Autodesk Inventor part; units mm, degrees
ref_plane "YZ Plane" through (0, 0, 0) normal (1, 0, 0) x (0, 1, 0)
ref_plane "XZ Plane" through (0, 0, 0) normal (0, 1, 0) x (-1, 0, 0)
ref_plane "XY Plane" through (0, 0, 0) normal (0, 0, 1) x (1, 0, 0)
sketch "sqr_sketch" plane through (0, 0, 0) normal (1, 0, 0) x (0, 1, 0)
  line L0 (12.7, 12.7) -> (-12.7, 12.7)
  line L1 (-12.7, 12.7) -> (-12.7, -12.7)
  line L2 (-12.7, -12.7) -> (12.7, -12.7)
  line L3 (12.7, -12.7) -> (12.7, 12.7)
  line L4 (12.7, 12.7) -> (-12.7, -12.7) construction
  line L5 (-12.7, 12.7) -> (12.7, -12.7) construction
  point P0 (0, 0)
  dimension "d0" = 25.4
extrude "sqr_extrusion" add sketch "sqr_sketch" along normal mid plane 25.4
sketch "T_sketch" plane through (-12.7, -12.7, 12.7) normal (0, 0, 1) x (1, 0, 0)
  line L0 (5.5534, 21.59) -> (19.8466, 21.59) construction
  line L1 (19.8466, 21.59) -> (19.8466, 3.81) construction
  line L2 (19.8466, 3.81) -> (5.5534, 3.81) construction
  line L3 (5.5534, 3.81) -> (5.5534, 21.59) construction
  line L4 (12.7, 21.59) -> (12.7, 3.81) construction
  line L5 (11.5041, 3.81) -> (11.5041, 19.4864)
  line L6 (11.5041, 19.4864) -> (5.539, 19.4864)
  line L7 (5.539, 19.4864) -> (5.539, 21.59)
  line L8 (5.539, 21.59) -> (19.8322, 21.59)
  line L9 (19.8322, 21.59) -> (19.8322, 19.4864)
  line L10 (19.8322, 19.4864) -> (13.8671, 19.4864)
  line L11 (13.8671, 19.4864) -> (13.8671, 3.81)
  line L12 (13.8671, 3.81) -> (11.5041, 3.81)
  point P0 (12.7, 12.7)
  point P1 (12.7, 12.7)
  point P2 (5.5534, 12.7)
  point P3 (19.8466, 12.7)
  dimension "d17" = 17.78
  dimension "d18" = 14.2932
extrude "T_extrusion" cut sketch "T_sketch" against normal blind 1
sketch "E_sketch" plane through (12.7, 0, 0) normal (1, 0, 0) x (0, 0, -1)
  line L0 (-6.8584, 8.89) -> (6.8584, 8.89) construction
  line L1 (6.8584, 8.89) -> (6.8584, -8.89) construction
  line L2 (6.8584, -8.89) -> (-6.8584, -8.89) construction
  line L3 (-6.8584, -8.89) -> (-6.8584, 8.89) construction
  line L4 (0, 8.89) -> (0, -8.89) construction
  line L5 (-5.0574, -8.89) -> (-5.0574, 8.89)
  line L6 (-5.0574, 8.89) -> (6.0659, 8.89)
  line L7 (6.0659, 8.89) -> (6.0659, 6.7864)
  line L8 (6.0659, 6.7864) -> (-2.6944, 6.7864)
  line L9 (-2.6944, 6.7864) -> (-2.6944, 1.9163)
  line L10 (-2.6944, 1.9163) -> (5.4752, 1.9163)
  line L11 (5.4752, 1.9163) -> (5.4752, -0.1873)
  line L12 (5.4752, -0.1873) -> (-2.6944, -0.1873)
  line L13 (-2.6944, -0.1873) -> (-2.6944, -6.7864)
  line L14 (-2.6944, -6.7864) -> (6.0659, -6.7864)
  line L15 (6.0659, -6.7864) -> (6.0659, -8.89)
  line L16 (6.0659, -8.89) -> (-5.0574, -8.89)
  point P0 (0, 0)
  point P1 (0, 0)
  point P2 (-6.8584, 0)
  point P3 (6.8584, 0)
  dimension "d15" = 17.78
  dimension "d16" = 13.7168
extrude "E_extrusion" cut sketch "E_sketch" against normal blind 1
sketch "A_sketch" plane through (12.7, 12.7, -12.7) normal (0, 0, -1) x (-1, 0, 0)
  line L0 (5.2508, -3.81) -> (20.1492, -3.81) construction
  line L1 (20.1492, -3.81) -> (20.1492, -21.59) construction
  line L2 (20.1492, -21.59) -> (5.2508, -21.59) construction
  line L3 (5.2508, -21.59) -> (5.2508, -3.81) construction
  line L4 (12.7, -3.81) -> (12.7, -21.59) construction
  line L5 (5.1356, -21.59) -> (11.1295, -3.81)
  line L6 (11.1295, -3.81) -> (14.04, -3.81)
  line L7 (14.04, -3.81) -> (20.0339, -21.59)
  line L8 (20.0339, -21.59) -> (17.5412, -21.59)
  line L9 (17.5412, -21.59) -> (15.9275, -16.6191)
  line L10 (15.9275, -16.6191) -> (9.1411, -16.6191)
  line L11 (9.1411, -16.6191) -> (7.5274, -21.59)
  line L12 (7.5274, -21.59) -> (5.1356, -21.59)
  line L13 (15.2791, -14.6019) -> (12.5271, -6.2306)
  line L14 (12.5271, -6.2306) -> (9.7895, -14.6019)
  line L15 (9.7895, -14.6019) -> (15.2791, -14.6019)
  point P0 (12.7, -12.7)
  point P1 (5.2508, -12.7)
  point P2 (20.1492, -12.7)
  point P3 (12.7, -12.7)
  dimension "d19" = 17.78
  dimension "d20" = 14.8983
extrude "A_extrusion" cut sketch "A_sketch" against normal blind 1
sketch "R_sketch" plane through (-12.7, 0, 0) normal (-1, 0, 0) x (0, 0, 1)
  line L0 (-7.586, 8.89) -> (7.586, 8.89) construction
  line L1 (7.586, 8.89) -> (7.586, -8.89) construction
  line L2 (7.586, -8.89) -> (-7.586, -8.89) construction
  line L3 (-7.586, -8.89) -> (-7.586, 8.89) construction
  line L4 (0, 8.89) -> (0, -8.89) construction
  line L5 (7.9751, -8.89) -> (4.9061, -8.89)
  line L6 (4.9061, -8.89) -> (-0.7132, -1.8155)
  line L7 (-0.7132, -1.8155) -> (-3.422, -1.8155)
  line L8 (-3.422, -1.8155) -> (-3.422, -8.89)
  line L9 (-3.422, -8.89) -> (-5.785, -8.89)
  line L10 (-5.785, -8.89) -> (-5.785, 8.89)
  line L11 (-5.785, 8.89) -> (-1.2031, 8.89)
  spline S0 degree 2 poles (-1.2031, 8.89) (0.3242, 8.89) (2.3846, 8.5586) (3.3211, 7.9535) knots 0 0 0 1 2 2 2
  spline S1 degree 2 poles (3.3211, 7.9535) (4.2577, 7.3483) (5.3383, 5.4608) (5.3383, 4.0632) knots 0 0 0 1 2 2 2
  spline S2 degree 2 poles (5.3383, 4.0632) (5.3383, 2.118) (3.35, -0.5187) (1.6498, -1.1527) knots 0 0 0 1 2 2 2
  line L12 (1.6498, -1.1527) -> (7.9751, -8.89)
  spline S3 degree 2 poles (2.8745, 3.8759) (2.8745, 4.6539) (2.327, 5.8498) (1.7506, 6.2388) knots 0 0 0 1 2 2 2
  spline S4 degree 2 poles (1.7506, 6.2388) (1.2463, 6.5702) (-0.0937, 6.844) (-1.0734, 6.844) knots 0 0 0 1 2 2 2
  line L13 (-1.0734, 6.844) -> (-3.422, 6.844)
  line L14 (-3.422, 6.844) -> (-3.422, 0.1585)
  line L15 (-3.422, 0.1585) -> (-1.3472, 0.1585)
  spline S5 degree 2 poles (-1.3472, 0.1585) (-0.3242, 0.1585) (1.304, 0.5187) (1.8659, 1.0806) knots 0 0 0 1 2 2 2
  spline S6 degree 2 poles (1.8659, 1.0806) (2.3846, 1.5705) (2.8745, 2.9537) (2.8745, 3.8759) knots 0 0 0 1 2 2 2
  point P0 (0, 0)
  point P1 (0, 0)
  point P2 (-7.586, 0)
  point P3 (7.586, 0)
  dimension "d21" = 17.78
  dimension "d22" = 15.1721
extrude "R_extrusion" cut sketch "R_sketch" against normal blind 1
sketch "C_sketch" plane through (-12.7, 12.7, 12.7) normal (0, 1, 0) x (1, 0, 0)
  line L0 (5.3589, 21.907) -> (20.0411, 21.907) construction
  line L1 (20.0411, 21.907) -> (20.0411, 3.493) construction
  line L2 (20.0411, 3.493) -> (5.3589, 3.493) construction
  line L3 (5.3589, 3.493) -> (5.3589, 21.907) construction
  line L4 (12.7, 21.907) -> (12.7, 3.493) construction
  spline S0 degree 2 poles (14.1048, 3.493) (12.3758, 3.493) (9.4509, 4.6601) (8.3847, 5.8272) knots 0 0 0 1 2 2 2
  spline S1 degree 2 poles (8.3847, 5.8272) (7.3185, 6.9799) (6.1514, 10.4379) (6.1514, 12.6856) knots 0 0 0 1 2 2 2
  spline S2 degree 2 poles (6.1514, 12.6856) (6.1514, 14.9189) (7.2896, 18.2328) (8.3703, 19.4576) knots 0 0 0 1 2 2 2
  spline S3 degree 2 poles (8.3703, 19.4576) (9.4365, 20.6535) (12.347, 21.907) (14.148, 21.907) knots 0 0 0 1 2 2 2
  spline S4 degree 2 poles (14.148, 21.907) (15.0414, 21.907) (16.6119, 21.6476) (17.2747, 21.4459) knots 0 0 0 1 2 2 2
  spline S5 degree 2 poles (17.2747, 21.4459) (17.851, 21.2586) (19.0469, 20.7255) (19.6377, 20.4085) knots 0 0 0 1 2 2 2
  line L5 (19.6377, 20.4085) -> (19.6377, 17.5556)
  line L6 (19.6377, 17.5556) -> (19.4503, 17.5556)
  spline S6 degree 2 poles (19.4503, 17.5556) (19.1334, 17.8438) (18.1536, 18.6507) (17.4476, 19.0397) knots 0 0 0 1 2 2 2
  spline S7 degree 2 poles (17.4476, 19.0397) (16.7704, 19.4143) (15.171, 19.8898) (14.1336, 19.8898) knots 0 0 0 1 2 2 2
  spline S8 degree 2 poles (14.1336, 19.8898) (12.9954, 19.8898) (10.9638, 18.9533) (10.2001, 18.0599) knots 0 0 0 1 2 2 2
  spline S9 degree 2 poles (10.2001, 18.0599) (9.4509, 17.1522) (8.6152, 14.4002) (8.6152, 12.6856) knots 0 0 0 1 2 2 2
  spline S10 degree 2 poles (8.6152, 12.6856) (8.6152, 10.8557) (9.4941, 8.219) (10.2578, 7.3112) knots 0 0 0 1 2 2 2
  spline S11 degree 2 poles (10.2578, 7.3112) (11.007, 6.4323) (13.0098, 5.539) (14.1336, 5.539) knots 0 0 0 1 2 2 2
  spline S12 degree 2 poles (14.1336, 5.539) (15.1566, 5.539) (16.9001, 6.0433) (17.5773, 6.4179) knots 0 0 0 1 2 2 2
  spline S13 degree 2 poles (17.5773, 6.4179) (18.2256, 6.7925) (19.191, 7.5706) (19.4648, 7.8444) knots 0 0 0 1 2 2 2
  line L7 (19.4648, 7.8444) -> (19.6377, 7.8444)
  line L8 (19.6377, 7.8444) -> (19.6377, 5.0203)
  spline S14 degree 2 poles (19.6377, 5.0203) (19.0469, 4.7465) (18.0095, 4.2423) (17.2747, 4.0117) knots 0 0 0 1 2 2 2
  spline S15 degree 2 poles (17.2747, 4.0117) (16.4966, 3.7524) (15.171, 3.493) (14.1048, 3.493) knots 0 0 0 1 2 2 2
  point P0 (12.7, 12.7)
  point P1 (5.3589, 12.7)
  point P2 (20.0411, 12.7)
  point P3 (12.7, 12.7)
  dimension "d23" = 18.414
  dimension "d24" = 14.6822
extrude "C_extrusion" cut sketch "C_sketch" against normal blind 1
sketch "I_sketch" plane through (-12.7, -12.7, -12.7) normal (0, -1, 0) x (1, 0, 0)
  line L0 (8.1397, 21.59) -> (17.2603, 21.59) construction
  line L1 (17.2603, 21.59) -> (17.2603, 3.81) construction
  line L2 (17.2603, 3.81) -> (8.1397, 3.81) construction
  line L3 (8.1397, 3.81) -> (8.1397, 21.59) construction
  line L4 (12.7, 3.81) -> (12.7, 21.59) construction
  line L5 (16.1364, 3.81) -> (9.2492, 3.81)
  line L6 (9.2492, 3.81) -> (9.2492, 5.6255)
  line L7 (9.2492, 5.6255) -> (11.5113, 5.6255)
  line L8 (11.5113, 5.6255) -> (11.5113, 19.7745)
  line L9 (11.5113, 19.7745) -> (9.2492, 19.7745)
  line L10 (9.2492, 19.7745) -> (9.2492, 21.59)
  line L11 (9.2492, 21.59) -> (16.1364, 21.59)
  line L12 (16.1364, 21.59) -> (16.1364, 19.7745)
  line L13 (16.1364, 19.7745) -> (13.8743, 19.7745)
  line L14 (13.8743, 19.7745) -> (13.8743, 5.6255)
  line L15 (13.8743, 5.6255) -> (16.1364, 5.6255)
  line L16 (16.1364, 5.6255) -> (16.1364, 3.81)
  point P0 (12.7, 12.7)
  point P1 (17.2603, 12.7)
  point P2 (8.1397, 12.7)
  point P3 (12.7, 12.7)
  dimension "d25" = 17.78
  dimension "d26" = 9.1205
extrude "I_extrusion" cut sketch "I_sketch" against normal blind 1
equation "\"d1\" = d0"
properties part number "Cubo" material "Rubber"
Input: part model. Units: mm. Frame: model coordinates. A direction names the side the tool comes from. Coordinates: 2 decimals unless noted, no trailing zeros.
1. Ray query, line 1 along X through (y, z) = (-8, 4.25); line 2 along X through (y, z) = (0, 4). Return the intervals inside material, ascending.
Checked values:
line 1: x = -11.7 to 11.7
line 2: x = -12.7 to 11.7
2. Access query for faces 3 (the flat face through (6.938, 12, -6)), 4 (the flat face through (4.6, -0.1, -12.2)), 5 (the flat face through (12, 1, -5.475)). Directions: +Z, -Z, +X, -X, +Y, -Y. A direction counts if a zero-diameter tool reaches every point of the face in a straight line with its end or side. Return the directions, or none.
Checked values:
face 3: +Y
face 4: -Z
face 5: +X
3. Draft query along Z for faces 1 (the flat face through (-12, 4, -3.422)), 2 (the flat face through (-4.295, 0.124, -12.207)). Return one class per face: +Z half, -Z half, draft (parallel to the pull), parting line (faces both ways), or undercut.
Checked values:
face 1: undercut
face 2: draft
